Design review of the part shown in the three views and the two pictorial views. Dimensions are in mm from the part's minimum x, y and z. A direction names the side the tool comes from. Coordinates: 2 decimals unless noted, no trailing zeros. Write each loop counter-clockwise with the first axis right and the second up, starting at its lowest first coordinate (ties: lowest second). Pieces come first, ordered by that corner, then holes. Notation, with made-up numbers: M -21,21 L 30,21 A22 cw 30,37 Z; hole C -20,-3 d9. An arc over 180 degrees is marked long. One line per question, with ' | ' between items.
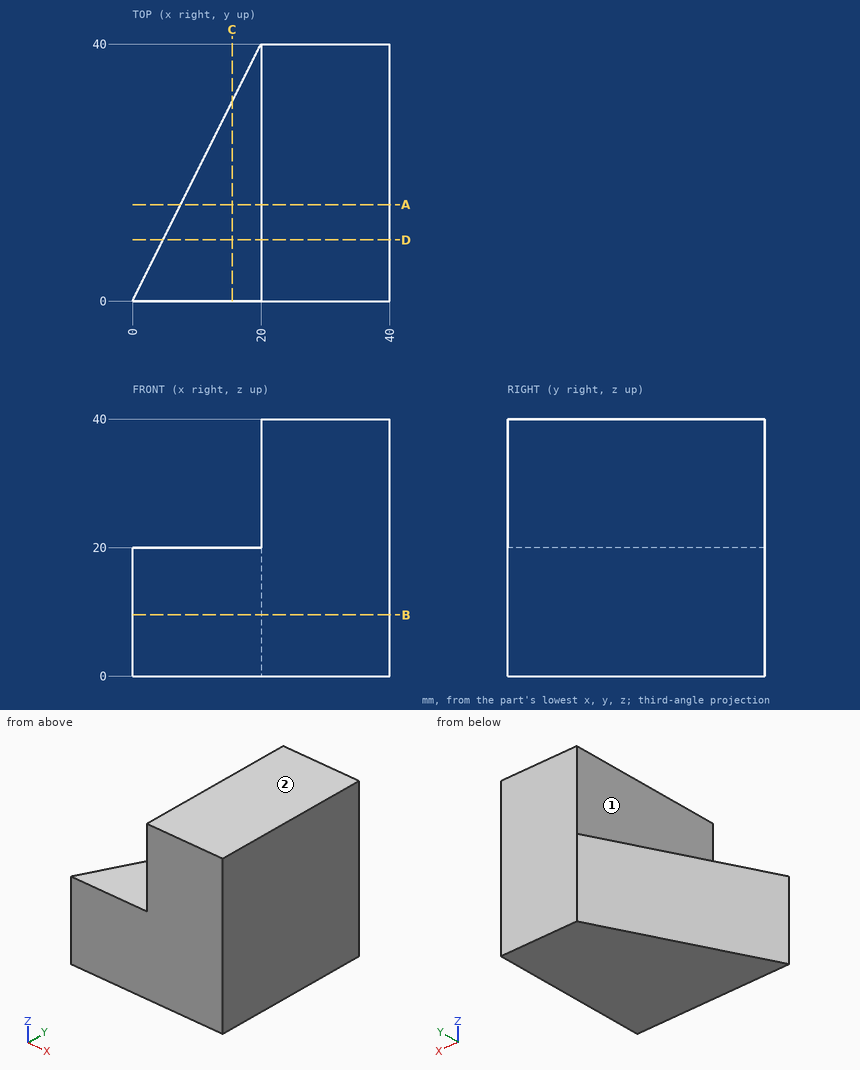
1. Machinability: for the marked faces 1 and 2, which of the approach directions +Z, -Z, +X, -X, +Y, -Y give a long, thin tool a straight path to every point of the face, cutting with its end or side? Answer none if there is none.
Computed values:
face 1: +Z, -X, +Y, -Y | face 2: +Z, +X, -X, +Y, -Y
2. Take a section at B-B on z = 9.5. State the section outline as (x, y) points.
Computed values:
outline: M 0,0 L 40,0 L 40,40 L 20,40 Z
3. Take a section at D-D on y = 9.5. State the section outline as (x, z) points, plus the area to 4 significant figures.
Computed values:
outline: M 4.75,0 L 40,0 L 40,40 L 20,40 L 20,20 L 4.75,20 Z | area: 1,105 mm2
4. For line 1 along X through (y, z) = (30, 32); line 2 along Z through (x, y) = (3.5, 3); line 3 along X through (y, z) = (29, 13.5), list the stretches that pass through material, from the lowest coordinate up.
Computed values:
line 1: x = 20 to 40 | line 2: z = 0 to 20 | line 3: x = 14.5 to 40
5. Take a section at C-C on x = 15.5. State the section outline as (y, z) points.
Computed values:
outline: M 0,0 L 31,0 L 31,20 L 0,20 Z
6. Take a section at A-A on y = 15. State the section outline as (x, z) points, plus the area to 3 significant figures.
Computed values:
outline: M 7.5,0 L 40,0 L 40,40 L 20,40 L 20,20 L 7.5,20 Z | area: 1,050 mm2
7. Clearance check with flat-ended pins moving along their axes: P1, Ø4, axis at x = 13.5, z = 7.5, coming from the +Y side; P2, Ø22, axis at x = 14.5, y = 14, coming from the +Z side; P3, Ø16, axis at y = 11, z = 32, coming from the -X side. State where each tip first meets the part, or that it passes through.
Computed values:
P1: stops at y = 31 | P2: stops at z = 40 | P3: stops at x = 20
